Could you check a few things on this model? Use its own coordinates, in mm. Give positions to 0.01 mm unless a question says otherwise; leave off trailing zeros. Loops run counter-clockwise (first coordinate to the right, second up) from the corner with the lowest first, then second, coordinate; pieces in that order, holes last. Notation, with made-up numbers: (-1.75, 83) -> (25.25, 83) arc R20 cw to (25.25, 107) -> close; hole circle Ø11 at (-4, 58). An arc over 180 degrees is marked (long way). Write item = value, one per line. Start each with the question number.
1) I want a section at B-B (z = 11.25). List the corners of the cut face in (x, y) for me.
2) I want a section at A-A (x = 33.5). List the corners of the cut face in (y, z) for me.
3) I want a section at C-C (z = 6.5). List the corners of the cut face in (x, y) for me, and give its area (3 significant figures).
4) I need wall thicknesses on probe 1 along Y at (x, z) = (34, 10.5); probe 2 along X at (y, z) = (9.75, 11.25); probe 3 along Y at (x, z) = (21.5, 7). Which ranges of each line are inside material? Lowest first, please. Write a range as from..to.
5) I'm going to push flat-ended pins straight in: pin 1 Ø1 at (y, z) = (4.5, 16.5) entering from +X; pin 2 Ø2.5 at (x, y) = (52, 9.5) entering from +Z; pin 3 Ø12 at (x, z) = (9, 8) entering from +Y; pin 4 Ø8 at (x, z) = (30.5, 4.5) entering from +Y. Where does each tip first touch, or does it pass through?
from build123d import *

# Parameters (mm, degrees)
F0_W        = 73
F0_H        = 20
F1_DEPTH    = 21
F2_W        = 3
F2_H        = 19
F3_DEPTH    = 73.001
F4_W        = 1.75
F4_H        = 3
F5_DEPTH    = 17
F6_R        = 1.74999
F7_T1_DEPTH = 72.9103913542
F7_T3_DEPTH = 72.9103913542
F9_DEPTH    = 20.001


# Not quite as in the source:
# - a fillet or chamfer that OpenCascade refuses, or shapes differently, is made with other operations: its cross-section is extruded or revolved along the edge and cut away or added
# - a fillet or chamfer is up to 0.001 mm smaller than in the source, because OpenCascade refuses the exact size


with BuildPart() as f1:
    # F0 (on Top) → F1 (new body)
    with BuildSketch(Plane.XY):
        with Locations((36.5, 10)):
            Rectangle(F0_W, F0_H)
    extrude(amount=F1_DEPTH)

    # F2 (on face) → F3 (cut, through all)
    with BuildSketch(Plane.YZ.offset(73)):
        Polygon((20, 21), (15.5, 21), (20, 0), align=None)
        with Locations((10, 11.5)):
            Rectangle(F2_W, F2_H)
        Polygon((4.5, 21), (0, 21), (0, 0), align=None)
    extrude(amount=-F3_DEPTH, mode=Mode.SUBTRACT)

    # F4 (on face) → F5 (join)
    with BuildSketch(Plane.XY.offset(2)):
        with Locations((35.625, 10)):
            Rectangle(F4_W, F4_H)
        with Locations((37.375, 10)):
            Rectangle(F4_W, F4_H)
    extrude(amount=F5_DEPTH)

    # F6 (radius 1.75 in the source; OpenCascade refuses exactly that, so slightly less here)
    f6_edges = [f1.edges().sort_by_distance(p)[0] for p in [
        (38.25, 10, 19),
        (34.75, 10, 19),
    ]]
    fillet(f6_edges, radius=F6_R)

    # F7: chamfer of 10 on 4 edges, made by hand

    # F7_s2 → F7_t1 (cut)
    with BuildSketch(Plane(origin=(0, -9.0103751492, 42.0484173631), x_dir=(1, 0, 0), z_dir=(0, 0.2095290887, -0.9778024141))):
        Polygon((73, -9.5560482815), (63, -19.5560482815), (73, -19.5560482815), align=None)
        Polygon((0, -9.5560482815), (10, -19.5560482815), (0, -19.5560482815), align=None)
    extrude(amount=F7_T1_DEPTH, mode=Mode.SUBTRACT)

    # F7_s4 → F7_t3 (cut)
    with BuildSketch(Plane(origin=(0, -5.3884239297, -25.1459783387), x_dir=(1, 0, 0), z_dir=(0, 0.2095290887, 0.9778024141))):
        Polygon((73, 10), (63, 0), (73, 0), align=None)
        Polygon((0, 10), (10, 0), (0, 0), align=None)
    extrude(amount=F7_T3_DEPTH, mode=Mode.SUBTRACT)

    # F8 (on Front) → F9 (cut, through all)
    with BuildSketch(Plane.XZ):
        Polygon((1.6886794803, 0), (6.0887903437, 21), (0, 21), (0, 0), align=None)
        Polygon((72.7780241408, 21), (66.9112096563, 21), (71.3113205197, 0), (72.7780241408, 0), align=None)
    extrude(amount=-F9_DEPTH, mode=Mode.SUBTRACT)


solid = f1.part
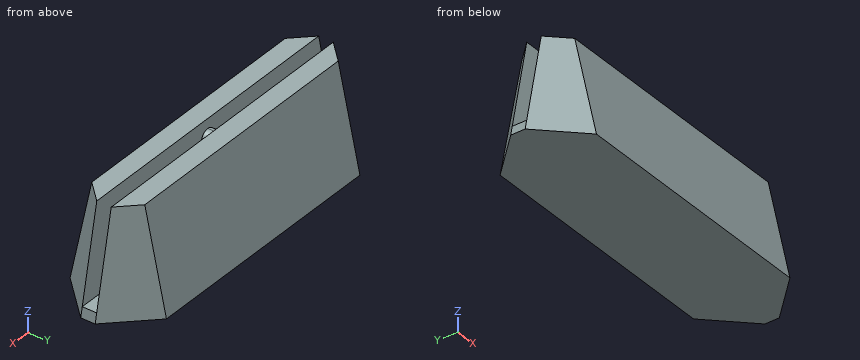
Answer list:
q1.outline = (4.05, 8.5) -> (10, 2.41) -> (63, 2.41) -> (68.95, 8.5) -> (38.25, 8.5) -> (38.25, 11.5) -> (68.95, 11.5) -> (63, 17.59) -> (10, 17.59) -> (4.05, 11.5) -> (34.75, 11.5) -> (34.75, 8.5) -> close
q2.outline = (0, 0) -> (20, 0) -> (15.5, 21) -> (11.5, 21) -> (11.5, 2) -> (8.5, 2) -> (8.5, 21) -> (4.5, 21) -> close
q3.outline = (3.05, 8.5) -> (10, 1.39) -> (63, 1.39) -> (69.95, 8.5) -> (38.25, 8.5) -> (38.25, 11.5) -> (69.95, 11.5) -> (63, 18.61) -> (10, 18.61) -> (3.05, 11.5) -> (34.75, 11.5) -> (34.75, 8.5) -> close
q3.area = 863 mm^2
q4.probe_1 = 2.25..8.5, 11.5..17.75
q4.probe_2 = 34.75..38.25
q4.probe_3 = 1.5..8.5, 11.5..18.5
q5.pin_1 = 64.44
q5.pin_2 = 21
q5.pin_3 = 19.55
q5.pin_4 = 19.89
